Autodesk Inventor part; units mm, degrees
ref_plane "YZ Plane" through (0, 0, 0) normal (1, 0, 0) x (0, 1, 0)
ref_plane "XZ Plane" through (0, 0, 0) normal (0, 1, 0) x (-1, 0, 0)
ref_plane "XY Plane" through (0, 0, 0) normal (0, 0, 1) x (1, 0, 0)
sketch "Эскиз1" plane through (0, 0, 0) normal (0, 1, 0) x (-1, 0, 0)
  line L0 (0, 0) -> (0, -20)
  circle A0 centre (0, -20) radius 2
  line L1 (-3.5, 25) -> (3.5, 25)
  line L2 (3.5, 25) -> (3.5, -25)
  line L3 (3.5, -25) -> (-3.5, -25)
  line L4 (-3.5, -25) -> (-3.5, 25)
  line L5 (-3.5, 25) -> (3.5, -25) construction
  line L6 (3.5, 25) -> (-3.5, -25) construction
  line L7 (0, 0) -> (0, 20)
  circle A1 centre (0, 20) radius 2
  dimension "d0" = 20
  dimension "d1" = 4
  dimension "d2" = 7
  dimension "d3" = 50
  dimension "d4" = 20
  dimension "d5" = 4
extrude "Выдавливание1" add sketch "Эскиз1" along normal blind 4 contours A0 | L1 L2 L3 L4 | A1
sketch "Эскиз2" plane through (3.5, 0, 25) normal (1, 0, 0) x (0, 0, -1)
  line L0 (50, 0) -> (0, 0)
  line L1 (0, 4) -> (50, 4)
  line L2 (50, 4) -> (50, 0)
  line L3 (50, 0) -> (0, 0)
  line L4 (0, 0) -> (0, 4)
  point P0 (25, 0)
extrude "Выдавливание2" add sketch "Эскиз2" along normal blind 7
sketch "Эскиз3" plane through (0, 4, 0) normal (0, 1, 0) x (1, 0, 0)
  line L0 (-3.5, -25) -> (10.5, -25)
  line L1 (-3.5, 25) -> (10.5, 25)
  line L2 (10.5, -25) -> (3.5, -25)
  line L3 (3.5, -25) -> (3.5, 25)
  line L4 (3.5, 25) -> (10.5, 25)
  line L5 (10.5, 25) -> (10.5, -25)
  point P0 (0, 0)
  dimension "d10" = 7
extrude "Выдавливание3" add sketch "Эскиз3" along normal blind 20
sketch "Эскиз5" plane through (0, 4, 0) normal (0, 1, 0) x (1, 0, 0)
  line L0 (-7.5352, -8.6362) -> (-7.5352, -8.5162)
  arc A0 (-1.7352, -8.5162) -> (-7.5352, -8.5162) centre (-4.6352, -8.5162) ccw
  line L1 (-1.7352, -8.5162) -> (-1.7352, -8.6362)
  arc A1 (1.3648, -12.5541) -> (-1.7352, -8.6362) centre (-4.6352, -14.1162) ccw
  line L2 (1.3648, -12.5541) -> (1.3648, 1.4338)
  arc A2 (1.3648, 1.4338) -> (0.6148, 2.1838) centre (0.6148, 1.4338) ccw
  line L3 (0.6148, 2.1838) -> (-9.8852, 2.1838)
  arc A3 (-9.8852, 2.1838) -> (-10.6352, 1.4338) centre (-9.8852, 1.4338) ccw
  line L4 (-10.6352, 1.4338) -> (-10.6352, -12.5541)
  arc A4 (-7.5352, -8.6362) -> (-10.6352, -12.5541) centre (-4.6352, -14.1162) ccw
  line L5 (0.4648, -4.2162) -> (0.4648, 0.7838)
  arc A5 (-0.0352, -4.7162) -> (0.4648, -4.2162) centre (-0.0352, -4.2162) ccw
  line L6 (-9.2352, -4.7162) -> (-0.0352, -4.7162)
  arc A6 (-9.7352, -4.2162) -> (-9.2352, -4.7162) centre (-9.2352, -4.2162) ccw
  line L7 (-9.7352, 0.7838) -> (-9.7352, -4.2162)
  arc A7 (-9.2352, 1.2838) -> (-9.7352, 0.7838) centre (-9.2352, 0.7838) ccw
  line L8 (-0.0352, 1.2838) -> (-9.2352, 1.2838)
  arc A8 (0.4648, 0.7838) -> (-0.0352, 1.2838) centre (-0.0352, 0.7838) ccw
  arc A9 (-5.1852, 5.8865) -> (-4.0852, 5.8865) centre (-4.6352, 4.9338) ccw
  line L9 (-5.1852, 7.0838) -> (-5.1852, 5.8865)
  line L10 (-5.1852, 7.0838) -> (-9.8852, 7.0838)
  arc A10 (-9.8852, 7.0838) -> (-10.7352, 6.2338) centre (-9.8852, 6.2338) ccw
  line L11 (-10.7352, 6.2338) -> (-10.7352, 1.4338)
  arc A11 (-9.8852, 2.2838) -> (-10.7352, 1.4338) centre (-9.8852, 1.4338) ccw
  line L12 (0.6148, 2.2838) -> (-9.8852, 2.2838)
  arc A12 (1.4648, 1.4338) -> (0.6148, 2.2838) centre (0.6148, 1.4338) ccw
  line L13 (1.4648, 1.4338) -> (1.4648, 6.2338)
  arc A13 (1.4648, 6.2338) -> (0.6148, 7.0838) centre (0.6148, 6.2338) ccw
  line L14 (0.6148, 7.0838) -> (-4.0852, 7.0838)
  line L15 (-4.0852, 5.8865) -> (-4.0852, 7.0838)
  line L16 (-9.8852, -25.0162) -> (-5.1852, -25.0162)
  line L17 (-5.1852, -23.8188) -> (-5.1852, -25.0162)
  arc A14 (-4.0852, -23.8188) -> (-5.1852, -23.8188) centre (-4.6352, -22.8662) ccw
  line L18 (-4.0852, -25.0162) -> (-4.0852, -23.8188)
  line L19 (-4.0852, -25.0162) -> (0.6148, -25.0162)
  arc A15 (0.6148, -25.0162) -> (1.4648, -24.1662) centre (0.6148, -24.1662) ccw
  line L20 (1.4648, -24.1662) -> (1.4648, -19.3662)
  arc A16 (0.6148, -20.2162) -> (1.4648, -19.3662) centre (0.6148, -19.3662) ccw
  line L21 (-9.8852, -20.2162) -> (0.6148, -20.2162)
  arc A17 (-10.7352, -19.3662) -> (-9.8852, -20.2162) centre (-9.8852, -19.3662) ccw
  line L22 (-10.7352, -19.3662) -> (-10.7352, -24.1662)
  arc A18 (-10.7352, -24.1662) -> (-9.8852, -25.0162) centre (-9.8852, -24.1662) ccw
  line L23 (-10.7352, -19.3662) -> (-10.7352, -15.6782)
  line L24 (-10.7352, -12.5541) -> (-10.7352, -14.1162)
  line L25 (-10.7352, -14.1162) -> (-10.7352, -15.6782)
  line L26 (-10.7352, -12.5541) -> (-10.7352, 1.4338)
  line L27 (1.4648, 1.4338) -> (1.4648, -12.5541)
  line L28 (1.4648, -15.6782) -> (1.4648, -19.3662)
  line L29 (1.4648, -15.6782) -> (1.4648, -14.1162)
  line L30 (1.4648, -14.1162) -> (1.4648, -12.5541)
  arc A19 (-10.6352, -15.6782) -> (-6.1972, -20.1162) centre (-4.6352, -14.1162) ccw
  line L31 (-10.6352, -15.6782) -> (-10.6352, -19.3662)
  arc A20 (-10.6352, -19.3662) -> (-9.8852, -20.1162) centre (-9.8852, -19.3662) ccw
  line L32 (-9.8852, -20.1162) -> (-6.1972, -20.1162)
  line L33 (1.3648, -19.3662) -> (1.3648, -15.6782)
  arc A21 (-3.0731, -20.1162) -> (1.3648, -15.6782) centre (-4.6352, -14.1162) ccw
  line L34 (-3.0731, -20.1162) -> (0.6148, -20.1162)
  arc A22 (0.6148, -20.1162) -> (1.3648, -19.3662) centre (0.6148, -19.3662) ccw
  circle A23 centre (-4.6352, 4.9338) radius 1.1
  line L35 (-5.1852, 5.8865) -> (-5.1852, 7.0838)
  line L36 (-4.0852, 7.0838) -> (-5.1852, 7.0838)
  circle A24 centre (-4.6352, -22.8662) radius 1.1
  line L37 (-5.1852, -25.0162) -> (-5.1852, -23.8188)
  line L38 (-4.0852, -25.0162) -> (-5.1852, -25.0162)
  circle A25 centre (-4.6352, -14.1162) radius 0.8
  line L39 (-3.5, 25) -> (3.5, 25)
  line L40 (-13.5, 25) -> (-13.5, -25)
  line L41 (-13.5, -25) -> (-3.5, -25)
  line L42 (-3.5, -25) -> (-3.5, 25)
  point P0 (0, 0)
  point P1 (-4.6352, -8.9662)
  dimension "d16" = 10
extrude "Выдавливание5" cut sketch "Эскиз5" against normal blind 10 contours A4 L4 A3 L3 L42 L8 A7 L7 A6 L6 A0 L0 | L0 A0 L42 L21 A17 L23 L25 L24 L26 A11 L12 L3 A3 L4 A4 | L42 L6 A5 L5 A8 L8 L3 A2 L2 A1 L1 A0 | A0 L1 A1 L2 A2 L3 L42 L12 A12 L27 L30 L29 L28 A16 L21 | L42 L8 A8 L5 A5 L6 | L6 A6 L7 A7 L8 L42 | A19 L32 A20 L31 | A22 L34 A21 L33 | A25
move faces "Перенос1" translate (-6.504, 0, 0) faces at (-3.5, 2.6667, -9.8559) (-3.5, 1.3333, 23.4054)
sketch "Эскиз6" plane through (0, 4, 0) normal (0, 1, 0) x (1, 0, 0)
  arc A0 (1.4648, -18.6645) -> (1.4648, -9.5679) centre (-2.6, -14.1162) ccw
  line L0 (1.4648, -9.5679) -> (1.4648, -19.3662)
  point P0 (0, 0)
  point P1 (0.2532, -8.7246)
  point P2 (-5.4532, -8.7246)
extrude "Выдавливание6" cut sketch "Эскиз6" against normal blind 7
sketch "Эскиз7" plane through (0, 0, 0) normal (0, -1, 0) x (1, 0, 0)
  line L0 (-10.004, 25) -> (-10.004, 20.2162)
  line L1 (-10.004, 21.4561) -> (4.0826, 21.4561)
  line L2 (4.0826, 21.4561) -> (4.0826, -3.0396)
  line L3 (4.0826, -3.0396) -> (-10.004, -3.0396)
  line L4 (-10.004, -3.0396) -> (-10.004, 21.4561)
  point P0 (0, 0)
extrude "Выдавливание7" cut sketch "Эскиз7" against normal blind 0.3
sketch "Эскиз8" plane through (0, 4, 0) normal (0, 1, 0) x (1, 0, 0)
  line L0 (-7.5352, -8.6362) -> (-7.5352, -8.5162)
  arc A0 (-1.7352, -8.5162) -> (-7.5352, -8.5162) centre (-4.6352, -8.5162) ccw
  line L1 (-1.7352, -8.5162) -> (-1.7352, -8.6362)
  arc A1 (1.3648, -12.5541) -> (-1.7352, -8.6362) centre (-4.6352, -14.1162) ccw
  line L2 (1.3648, -12.5541) -> (1.3648, 1.4338)
  arc A2 (1.3648, 1.4338) -> (0.6148, 2.1838) centre (0.6148, 1.4338) ccw
  line L3 (0.6148, 2.1838) -> (-9.8852, 2.1838)
  arc A3 (-9.8852, 2.1838) -> (-10.6352, 1.4338) centre (-9.8852, 1.4338) ccw
  line L4 (-10.6352, 1.4338) -> (-10.6352, -12.5541)
  arc A4 (-7.5352, -8.6362) -> (-10.6352, -12.5541) centre (-4.6352, -14.1162) ccw
  line L5 (0.4648, -4.2162) -> (0.4648, 0.7838)
  arc A5 (-0.0352, -4.7162) -> (0.4648, -4.2162) centre (-0.0352, -4.2162) ccw
  line L6 (-9.2352, -4.7162) -> (-0.0352, -4.7162)
  arc A6 (-9.7352, -4.2162) -> (-9.2352, -4.7162) centre (-9.2352, -4.2162) ccw
  line L7 (-9.7352, 0.7838) -> (-9.7352, -4.2162)
  arc A7 (-9.2352, 1.2838) -> (-9.7352, 0.7838) centre (-9.2352, 0.7838) ccw
  line L8 (-0.0352, 1.2838) -> (-9.2352, 1.2838)
  arc A8 (0.4648, 0.7838) -> (-0.0352, 1.2838) centre (-0.0352, 0.7838) ccw
  arc A9 (-5.1852, 5.8865) -> (-4.0852, 5.8865) centre (-4.6352, 4.9338) ccw
  line L9 (-5.1852, 7.0838) -> (-5.1852, 5.8865)
  line L10 (-5.1852, 7.0838) -> (-9.8852, 7.0838)
  arc A10 (-9.8852, 7.0838) -> (-10.7352, 6.2338) centre (-9.8852, 6.2338) ccw
  line L11 (-10.7352, 6.2338) -> (-10.7352, 1.4338)
  arc A11 (-9.8852, 2.2838) -> (-10.7352, 1.4338) centre (-9.8852, 1.4338) ccw
  line L12 (0.6148, 2.2838) -> (-9.8852, 2.2838)
  arc A12 (1.4648, 1.4338) -> (0.6148, 2.2838) centre (0.6148, 1.4338) ccw
  line L13 (1.4648, 1.4338) -> (1.4648, 6.2338)
  arc A13 (1.4648, 6.2338) -> (0.6148, 7.0838) centre (0.6148, 6.2338) ccw
  line L14 (0.6148, 7.0838) -> (-4.0852, 7.0838)
  line L15 (-4.0852, 5.8865) -> (-4.0852, 7.0838)
  line L16 (-9.8852, -25.0162) -> (-5.1852, -25.0162)
  line L17 (-5.1852, -23.8188) -> (-5.1852, -25.0162)
  arc A14 (-4.0852, -23.8188) -> (-5.1852, -23.8188) centre (-4.6352, -22.8662) ccw
  line L18 (-4.0852, -25.0162) -> (-4.0852, -23.8188)
  line L19 (-4.0852, -25.0162) -> (0.6148, -25.0162)
  arc A15 (0.6148, -25.0162) -> (1.4648, -24.1662) centre (0.6148, -24.1662) ccw
  line L20 (1.4648, -24.1662) -> (1.4648, -19.3662)
  arc A16 (0.6148, -20.2162) -> (1.4648, -19.3662) centre (0.6148, -19.3662) ccw
  line L21 (-9.8852, -20.2162) -> (0.6148, -20.2162)
  arc A17 (-10.7352, -19.3662) -> (-9.8852, -20.2162) centre (-9.8852, -19.3662) ccw
  line L22 (-10.7352, -19.3662) -> (-10.7352, -24.1662)
  arc A18 (-10.7352, -24.1662) -> (-9.8852, -25.0162) centre (-9.8852, -24.1662) ccw
  line L23 (-10.7352, -19.3662) -> (-10.7352, -15.6782)
  line L24 (-10.7352, -12.5541) -> (-10.7352, -14.1162)
  line L25 (-10.7352, -14.1162) -> (-10.7352, -15.6782)
  line L26 (-10.7352, -12.5541) -> (-10.7352, 1.4338)
  line L27 (1.4648, 1.4338) -> (1.4648, -12.5541)
  line L28 (1.4648, -15.6782) -> (1.4648, -19.3662)
  line L29 (1.4648, -15.6782) -> (1.4648, -14.1162)
  line L30 (1.4648, -14.1162) -> (1.4648, -12.5541)
  arc A19 (-10.6352, -15.6782) -> (-6.1972, -20.1162) centre (-4.6352, -14.1162) ccw
  line L31 (-10.6352, -15.6782) -> (-10.6352, -19.3662)
  arc A20 (-10.6352, -19.3662) -> (-9.8852, -20.1162) centre (-9.8852, -19.3662) ccw
  line L32 (-9.8852, -20.1162) -> (-6.1972, -20.1162)
  line L33 (1.3648, -19.3662) -> (1.3648, -15.6782)
  arc A21 (-3.0731, -20.1162) -> (1.3648, -15.6782) centre (-4.6352, -14.1162) ccw
  line L34 (-3.0731, -20.1162) -> (0.6148, -20.1162)
  arc A22 (0.6148, -20.1162) -> (1.3648, -19.3662) centre (0.6148, -19.3662) ccw
  circle A23 centre (-4.6352, 4.9338) radius 1.1
  line L35 (-5.1852, 5.8865) -> (-5.1852, 7.0838)
  line L36 (-4.0852, 7.0838) -> (-5.1852, 7.0838)
  circle A24 centre (-4.6352, -22.8662) radius 1.1
  line L37 (-5.1852, -25.0162) -> (-5.1852, -23.8188)
  line L38 (-4.0852, -25.0162) -> (-5.1852, -25.0162)
  circle A25 centre (-4.6352, -14.1162) radius 0.8
  line L39 (-3.5, 25) -> (3.5, 25)
  line L40 (-13.5, 25) -> (-13.5, -25)
  line L41 (-13.5, -25) -> (-3.5, -25)
  line L42 (-3.5, -25) -> (-3.5, 25)
  point P0 (0, 0)
  point P1 (0, 0)
  point P2 (-4.6352, -8.9662)
  dimension "d26" = 10
extrude "Выдавливание8" cut sketch "Эскиз8" against normal through all contours A24 A14 | A9 A23
move faces "Перенос2" translate (-2.5, 0, 0) faces at (10.5, 8, -8.3333)
chamfer "Фаска1" distance 2 angle 45 2 edges at (3.5, 14, 25) (3.5, 14, -25)
properties part number "000.705 - Пассивный прижим"
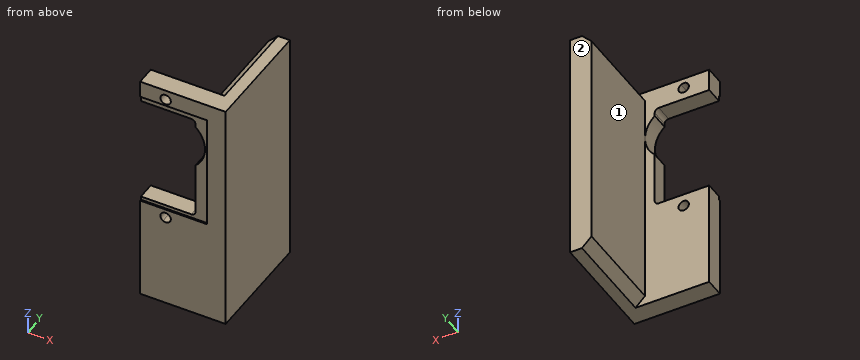
Can you work these out from the model? Positions are in its coordinate system, mm. Face numbers are marked on the shaded views. A direction names the side the tool comes from. Give positions to 0.01 mm unless a question says otherwise; leave off trailing zeros. Order: outer loops, then holes, each group sorted by start corner. A loop starts at its lowest first (then second) coordinate and runs counter-clockwise, first axis right, second up. Notation, with made-up numbers: M -15.75,47 L 41.25,47 A16 cw 41.25,74 Z; hole C 67.5,50 d6. An arc over 180 degrees is marked long. Use one line per item in the form item = value.
Item 1: If we section it at C-C, the plane y = 18.75: Write out the boundary of the cut face in (x, z).
Values follow:
outline = M 3.5,-23 L 5.5,-25 L 8,-25 L 8,25 L 5.5,25 L 3.5,23 Z
Item 2: If we section it at B-B, the plane z = 3.5: Write out the boundary of the cut face in (x, y), and give its area (3 significant figures).
Values follow:
outline = M 1.46,0.3 L 4.08,0.3 L 4.08,0 L 8,0 L 8,24 L 3.5,24 L 3.5,4 L 1.46,4 Z
area = 115 mm^2
Item 3: If we section it at D-D, the plane y = 3.5: Write out the boundary of the cut face in (x, z).
Values follow:
outline = M -10,-25 L 8,-25 L 8,25 L -10,25 L -10,20.22 L 0.61,20.22 A0.85 cw 1.46,19.37 L 1.46,18.66 A6.1 cw 1.46,9.57 L 1.46,-1.43 A0.85 cw 0.61,-2.28 L -10,-2.28 Z; hole C -4.64,-4.93 d2.2; hole M -5.19,23.82 A1.1 ccw long -4.09,23.82 A1.1 ccw Z
Item 4: If we section it at A-A, the plane x = -1.75: Write out the boundary of the cut face in (y, z), and give its area (3 significant figures).
Values follow:
outline = M 0,-25 L 4,-25 L 4,-2.28 L 0.3,-2.28 L 0.3,-3.04 L 0,-3.04 Z; M 0,21.46 L 0.3,21.46 L 0.3,20.22 L 4,20.22 L 4,25 L 0,25 Z
area = 109 mm^2
Item 5: If I drill on line 1 along Y through (x, z) = (1.5, -23); line 2 along X through (y, z) = (21.5, -10.5); line 3 along Z through (x, y) = (2.25, 1.75), over which ranges is the centre line in solid material (lowest first)? Write a range as [from, to].
Values follow:
line_1 = [0, 4]
line_2 = [3.5, 8]
line_3 = [-25, 10.42], [17.82, 25]
Item 6: Will these pins go through, and if not, where does the flat tip stop? pin 1 Ø1.5 at (x, z) = (0.5, -14) entering from -Y; pin 2 Ø5 at (y, z) = (10, -2.5) entering from -X; pin 3 Ø8.5 at (x, z) = (-2, 19.5) entering from +Y; pin 4 Ø8 at (x, y) = (0, 17.5) entering from +Z.
Values follow:
pin_1 = 0
pin_2 = 3.5
pin_3 = 4
pin_4 = 23.5
Item 7: For the marked faces 1 and 2, which set-ups out of +Z, -Z, +X, -X, +Y, -Y let a thin tool reach every point of the face, with its end or its side?
Values follow:
face_1 = +Z, -Z, -X, +Y
face_2 = +Z, -Z, +X, -X, +Y
